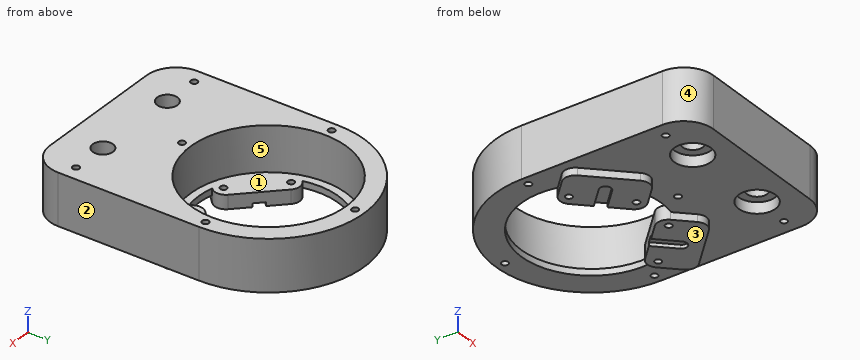
from build123d import *

# Parameters (mm, degrees)
SKETCH_2_R                  = 19
SKETCH_2_R_2                = 2.75
EXTRUDE_1_DEPTH             = 13.9
SKETCH_3_R                  = 21.125
CUT_EXTRUDE_1_DEPTH         = 12.15
SKETCH_4_R                  = 5
CUT_EXTRUDE_2_DEPTH         = 3
FILLET_1_R                  = 8
SKETCH_5_R                  = 0.9
CUT_EXTRUDE_3_DEPTH         = 60.993937194
SKETCH_6_R                  = 0.9
EXTRUDE_2_DEPTH             = 2
EXTRUDE_2_DIRECTION_2_REACH = 61.994
CUT_EXTRUDE_4_DEPTH         = 1


with BuildPart() as part:
    # Sketch 2 → Extrude 1 (new body)
    with BuildSketch(Plane.XY):
        with BuildLine():
            ThreePointArc((26, 26.25), (0, 52.25), (-26, 26.25))
            Line((-26, 26.25), (-26, -20))
            Line((-26, -20), (26, -20))
            Line((26, -20), (26, 26.25))
        make_face()
        with Locations((0, 26.25)):
            Circle(SKETCH_2_R, mode=Mode.SUBTRACT)
        with Locations((12, -10)):
            Circle(SKETCH_2_R_2, mode=Mode.SUBTRACT)
        with Locations((-12, -10)):
            Circle(SKETCH_2_R_2, mode=Mode.SUBTRACT)
    extrude(amount=EXTRUDE_1_DEPTH)

    # Sketch 3 → Cut-Extrude 1 (cut)
    with BuildSketch(Plane.XY.offset(13.9)):
        with Locations((0, 26.25)):
            Circle(SKETCH_3_R)
    extrude(amount=-CUT_EXTRUDE_1_DEPTH, mode=Mode.SUBTRACT)

    # Sketch 4 → Cut-Extrude 2 (cut)
    with BuildSketch(Plane(origin=(0, 0, 0), x_dir=(-1, 0, 0), z_dir=(0, 0, -1))):
        with Locations((-12, -10)):
            Circle(SKETCH_4_R)
        with Locations((12, -10)):
            Circle(SKETCH_4_R)
    extrude(amount=-CUT_EXTRUDE_2_DEPTH, mode=Mode.SUBTRACT)

    # Fillet 1
    fillet_1_edges = [part.edges().sort_by_distance(p)[0] for p in [
        (26, -20, 6.95),
        (-26, -20, 6.95),
    ]]
    fillet(fillet_1_edges, radius=FILLET_1_R)

    # Sketch 5 → Cut-Extrude 3 (cut, through all)
    with BuildSketch(Plane.XY.offset(13.9)):
        with Locations((0, 49.75)):
            Circle(SKETCH_5_R)
        with Locations((-23.5, 26.25)):
            Circle(SKETCH_5_R)
        with Locations((0, 2.75)):
            Circle(SKETCH_5_R)
        with Locations((23.5, 26.25)):
            Circle(SKETCH_5_R)
        with Locations((-22, -10)):
            Circle(SKETCH_5_R)
        with Locations(Location((22, -10, 0), (0, 0, 180))):
            Circle(SKETCH_5_R)
    extrude(amount=-CUT_EXTRUDE_3_DEPTH, mode=Mode.SUBTRACT)

    # Sketch 6 → Extrude 2 (add)
    # profile 1 of 2: a face of its own
    with BuildSketch(Plane(origin=(0, 0, 0), x_dir=(-1, 0, 0), z_dir=(0, 0, -1))):
        with BuildLine():
            Line((-22.627416998, 17.764718626), (-18.384776311, 22.007359313))
            ThreePointArc((-18.384776311, 22.007359313), (-16.263455967, 22.886038969), (-14.142135624, 22.007359313))
            Line((-14.142135624, 22.007359313), (-4.242640687, 12.107864376))
            ThreePointArc((-4.242640687, 12.107864376), (-3.363961031, 9.986544033), (-4.242640687, 7.865223689))
            Line((-4.242640687, 7.865223689), (-8.485281374, 3.622583002))
            ThreePointArc((-8.485281374, 3.622583002), (-10.606601718, 2.743903346), (-12.727922061, 3.622583002))
            Line((-12.727922061, 3.622583002), (-22.627416998, 13.522077939))
            ThreePointArc((-22.627416998, 13.522077939), (-23.506096654, 15.643398282), (-22.627416998, 17.764718626))
        make_face()
        with Locations((-16.617009358, 20.23959236)):
            Circle(SKETCH_6_R, mode=Mode.SUBTRACT)
        with Locations((-6.01040764, 9.632990642)):
            Circle(SKETCH_6_R, mode=Mode.SUBTRACT)
    # profile 2 of 2: a face of its own
    with BuildSketch(Plane(origin=(0, 0, 0), x_dir=(-1, 0, 0), z_dir=(0, 0, -1))):
        with BuildLine():
            Line((14.142135624, 22.007359313), (4.242640687, 12.107864376))
            ThreePointArc((4.242640687, 12.107864376), (3.363961031, 9.986544033), (4.242640687, 7.865223689))
            Line((4.242640687, 7.865223689), (8.485281374, 3.622583002))
            ThreePointArc((8.485281374, 3.622583002), (10.606601718, 2.743903346), (12.727922061, 3.622583002))
            Line((12.727922061, 3.622583002), (22.627416998, 13.522077939))
            ThreePointArc((22.627416998, 13.522077939), (23.506096654, 15.643398282), (22.627416998, 17.764718626))
            Line((22.627416998, 17.764718626), (18.384776311, 22.007359313))
            ThreePointArc((18.384776311, 22.007359313), (16.263455967, 22.886038969), (14.142135624, 22.007359313))
        make_face()
        with Locations(Location((6.01040764, 9.632990642, 0), (0, 0, 180))):
            Circle(SKETCH_6_R, mode=Mode.SUBTRACT)
        with Locations(Location((16.617009358, 20.23959236, 0), (0, 0, 180))):
            Circle(SKETCH_6_R, mode=Mode.SUBTRACT)
    extrude(amount=EXTRUDE_2_DEPTH)

    # Extrude 2 direction 2: up to this face of the body (flat: up to its plane)
    extrude_2_direction_2_end = Plane(part.part.faces().sort_by_distance((-20.52749477, 26.25, 1.75))[0])
    # Sketch 6 → Extrude 2 direction 2 (add, up to the picked face)
    with BuildSketch(Plane(origin=(0, 0, 0), x_dir=(-1, 0, 0), z_dir=(0, 0, -1)), mode=Mode.PRIVATE) as extrude_2_direction_2_sk1:
        with BuildLine():
            Line((-22.627416998, 17.764718626), (-18.384776311, 22.007359313))
            ThreePointArc((-18.384776311, 22.007359313), (-16.263455967, 22.886038969), (-14.142135624, 22.007359313))
            Line((-14.142135624, 22.007359313), (-4.242640687, 12.107864376))
            ThreePointArc((-4.242640687, 12.107864376), (-3.363961031, 9.986544033), (-4.242640687, 7.865223689))
            Line((-4.242640687, 7.865223689), (-8.485281374, 3.622583002))
            ThreePointArc((-8.485281374, 3.622583002), (-10.606601718, 2.743903346), (-12.727922061, 3.622583002))
            Line((-12.727922061, 3.622583002), (-22.627416998, 13.522077939))
            ThreePointArc((-22.627416998, 13.522077939), (-23.506096654, 15.643398282), (-22.627416998, 17.764718626))
        make_face()
        with Locations((-16.617009358, 20.23959236)):
            Circle(SKETCH_6_R, mode=Mode.SUBTRACT)
        with Locations((-6.01040764, 9.632990642)):
            Circle(SKETCH_6_R, mode=Mode.SUBTRACT)
    extrude_2_direction_2_tool1 = split(extrude(extrude_2_direction_2_sk1.sketch, amount=-EXTRUDE_2_DIRECTION_2_REACH, mode=Mode.PRIVATE), bisect_by=extrude_2_direction_2_end, keep=Keep.BOTH, mode=Mode.PRIVATE)
    # Sketch 6 → Extrude 2 direction 2 (add, up to the picked face)
    with BuildSketch(Plane(origin=(0, 0, 0), x_dir=(-1, 0, 0), z_dir=(0, 0, -1)), mode=Mode.PRIVATE) as extrude_2_direction_2_sk2:
        with BuildLine():
            Line((14.142135624, 22.007359313), (4.242640687, 12.107864376))
            ThreePointArc((4.242640687, 12.107864376), (3.363961031, 9.986544033), (4.242640687, 7.865223689))
            Line((4.242640687, 7.865223689), (8.485281374, 3.622583002))
            ThreePointArc((8.485281374, 3.622583002), (10.606601718, 2.743903346), (12.727922061, 3.622583002))
            Line((12.727922061, 3.622583002), (22.627416998, 13.522077939))
            ThreePointArc((22.627416998, 13.522077939), (23.506096654, 15.643398282), (22.627416998, 17.764718626))
            Line((22.627416998, 17.764718626), (18.384776311, 22.007359313))
            ThreePointArc((18.384776311, 22.007359313), (16.263455967, 22.886038969), (14.142135624, 22.007359313))
        make_face()
        with Locations(Location((6.01040764, 9.632990642, 0), (0, 0, 180))):
            Circle(SKETCH_6_R, mode=Mode.SUBTRACT)
        with Locations(Location((16.617009358, 20.23959236, 0), (0, 0, 180))):
            Circle(SKETCH_6_R, mode=Mode.SUBTRACT)
    extrude_2_direction_2_tool2 = split(extrude(extrude_2_direction_2_sk2.sketch, amount=-EXTRUDE_2_DIRECTION_2_REACH, mode=Mode.PRIVATE), bisect_by=extrude_2_direction_2_end, keep=Keep.BOTH, mode=Mode.PRIVATE)
    add(extrude_2_direction_2_tool1.solids().sort_by(Axis((13.48255, 12.76745, 0), (0, 0, 1)))[0])
    add(extrude_2_direction_2_tool2.solids().sort_by(Axis((-13.48255, 12.76745, 0), (0, 0, 1)))[0])

    # Sketch 7 → Cut-Extrude 4 (cut)
    with BuildSketch(Plane(origin=(0, 0, -2), x_dir=(-1, 0, 0), z_dir=(0, 0, -1))):
        with BuildLine():
            Line((-15.202795796, 13.168524548), (-10.253048327, 18.118272016))
            ThreePointArc((-10.253048327, 18.118272016), (-8.131727984, 18.118272016), (-8.131727984, 15.996951673))
            Line((-8.131727984, 15.996951673), (-13.081475452, 11.047204204))
            ThreePointArc((-13.081475452, 11.047204204), (-15.202795796, 11.047204204), (-15.202795796, 13.168524548))
        make_face()
        with BuildLine():
            Line((15.202795796, 13.168524548), (10.253048327, 18.118272016))
            ThreePointArc((10.253048327, 18.118272016), (8.131727984, 18.118272016), (8.131727984, 15.996951673))
            Line((8.131727984, 15.996951673), (13.081475452, 11.047204204))
            ThreePointArc((13.081475452, 11.047204204), (15.202795796, 11.047204204), (15.202795796, 13.168524548))
        make_face()
    extrude(amount=-CUT_EXTRUDE_4_DEPTH, mode=Mode.SUBTRACT)


solid = part.part
Design review of the part built by this model. Coordinates are the model's own, in mm. Face numbers are marked on the shaded views. A direction names the side the tool comes from. Give positions to 0.01 mm unless a question says otherwise; leave off trailing zeros. Loops run counter-clockwise (first coordinate to the right, second up) from the corner with the lowest first, then second, coordinate; pieces in that order, holes last. Notation, with made-up numbers: M 36.25,-28.5 L 58.25,-28.5 A23 cw 58.25,-6.5 Z; hole C 22.25,-5 d9. An arc over 180 degrees is marked long. Answer as a JSON object with one key per item and string values.
Item 1: Mouldability with a two-part tool opening along X and no side actions: class the marked faces 1, 2 and 3 as pulls with the +X half, pulls with the -X half, needs draft (parallel to the pull), parting line crosses it, or undercut.
Output values:
{"face 1": "undercut", "face 2": "pulls with the +X half", "face 3": "needs draft"}
Item 2: We need section D-D (x = -12). State the section outline as (y, z) points, and give its area (3 significant figures).
Output values:
{"outline": "M -20,0 L -15,0 L -15,3 L -12.75,3 L -12.75,13.9 L -20,13.9 Z; M -7.25,3 L -5,3 L -5,0 L 3.09,0 L 3.09,-2 L 12.13,-2 L 12.13,-1 L 16.37,-1 L 16.37,-2 L 19.87,-2 L 19.87,1.75 L 8.86,1.75 L 8.86,13.9 L -7.25,13.9 Z; M 40.98,0 L 49.32,0 L 49.32,13.9 L 43.64,13.9 L 43.64,1.75 L 40.98,1.75 Z", "area": "443 mm2"}
Item 3: For P1, Ø2.5, axis at x = 0, y = 2.75, coming from the -Z side; P2, Ø3, axis at x = -19, z = 5, coming from the +Y side; P3, Ø1.5, axis at y = 43, z = -0.5, coming from the -X side; P4, Ø1.4, axis at x = -16.62, y = 20.24, coming from the -Z side, all flat-tipped, find the tip position at first contact; note any pin that passes through.
Output values:
{"P1": "stops at z = 0", "P2": "stops at y = 45.48", "P3": "stops at x = -20.34", "P4": "passes through"}
Item 4: Machinability: for the marked faces 4 and 5, which of the approach directions +Z, -Z, +X, -X, +Y, -Y give a long, thin tool a straight path to every point of the face, cutting with its end or side? Answer none if there is none.
Output values:
{"face 4": "+Z, -Z, -X, -Y", "face 5": "+Z"}
Item 5: We need section B-B (x = 0). State the section outline as (y, z) points (3 decimals), and give its area (3 significant figures).
Output values:
{"outline": "M -20,0 L 1.85,0 L 1.85,13.9 L -20,13.9 Z; M 3.65,0 L 7.25,0 L 7.25,1.75 L 5.125,1.75 L 5.125,13.9 L 3.65,13.9 Z; M 45.25,0 L 48.85,0 L 48.85,13.9 L 47.375,13.9 L 47.375,1.75 L 45.25,1.75 Z; M 50.65,0 L 52.25,0 L 52.25,13.9 L 50.65,13.9 Z", "area": "374 mm2"}
Item 6: We need section A-A (y = -10). State the section outline as (x, z) points, and give its area (3 significant figures).
Output values:
{"outline": "M -26,0 L -22.9,0 L -22.9,13.9 L -26,13.9 Z; M -21.1,0 L -17,0 L -17,3 L -14.75,3 L -14.75,13.9 L -21.1,13.9 Z; M -9.25,3 L -7,3 L -7,0 L 7,0 L 7,3 L 9.25,3 L 9.25,13.9 L -9.25,13.9 Z; M 14.75,3 L 17,3 L 17,0 L 21.1,0 L 21.1,13.9 L 14.75,13.9 Z; M 22.9,0 L 26,0 L 26,13.9 L 22.9,13.9 Z", "area": "493 mm2"}
Item 7: We need section C-C (z = 12.25). Count the separate pieces of the cut face and the enclosed holes in it, and give its area (3 significant figures).
Output values:
{"separate pieces": "1", "enclosed holes": "9", "area": "1,970 mm2"}
Item 8: Wall thickness on line 1 along Y through (x, z) = (-14, 2.25); line 2 along Y through (x, z) = (12.5, 11); line 3 along Y through (x, z) = (-6, 5.75): over which ranges is each line inside the solid? List them lowest first.
Output values:
{"line 1": "y = -20 to -14.58, -5.42 to 10.43, 42.07 to 48.16", "line 2": "y = -20 to -12.7, -7.3 to 9.22, 43.28 to 49.05", "line 3": "y = -20 to 5.99, 46.51 to 51.55"}
